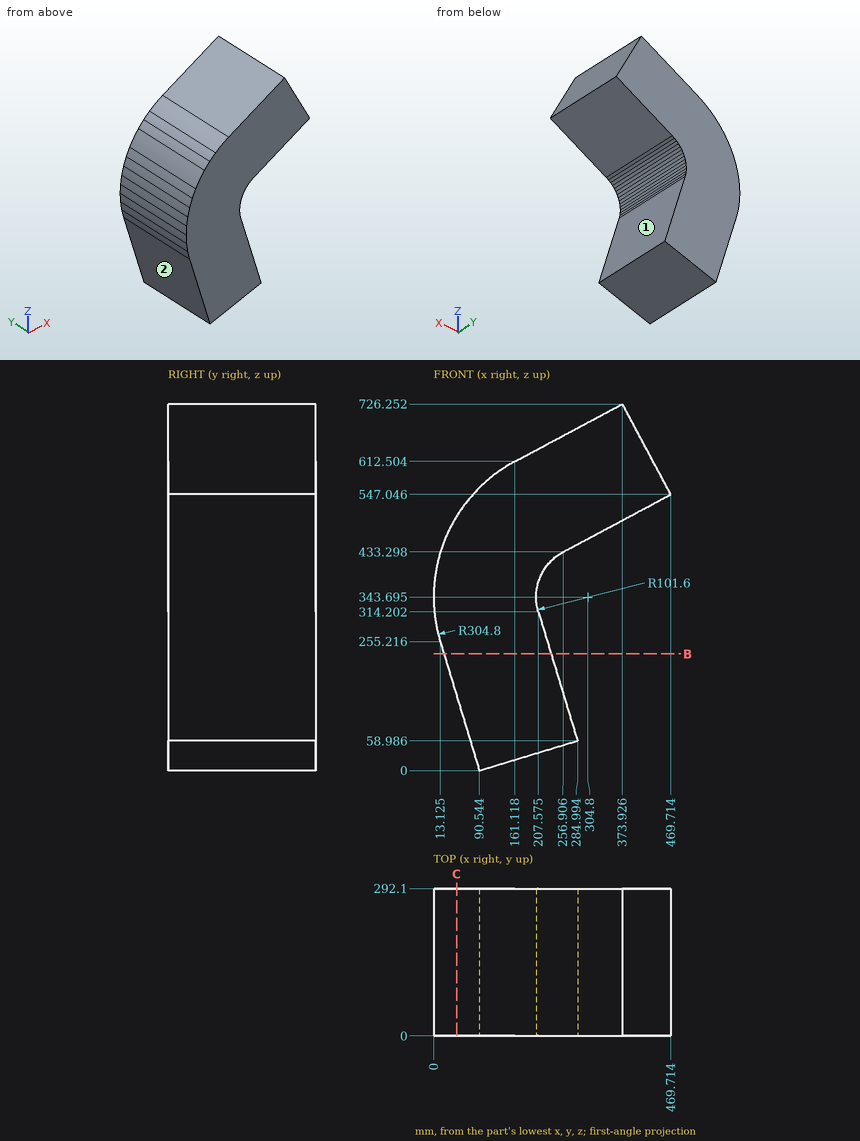
Check sheet for the drawn part. Datum: minimum x, y, z corner. Units: mm. A direction names the side the tool comes from. Round coordinates to 2 decimals unless told otherwise and drop trailing zeros. Loops run counter-clockwise (first coordinate to the right, second up) from the corner with the lowest first, then second, coordinate; pieces in that order, holes last. Notation, with made-up numbers: (88, 21) -> (114, 21) arc R25 ccw to (114, 39) -> close; hole circle Ø5 at (31, -30.75). An arc over 180 degrees is marked (long way). Put each result on its own line as item: value. Start each with the question number.
1. Access from +Z, -Z, +X, -X, +Y, -Y to the whole of each face (thin tool, end or side, straight path). Record for the marked faces 1 and 2.
2. Section check C-C (x = 45.5). Enter the section's corners in (y, z), plus the area to 3 significant figures.
3. Scan lines: probe 1 along X at (y, z) = (205, 216) (1 decimal); probe 2 along X at (y, z) = (121, 127.5); probe 3 along Z at (x, y) = (165.5, 125.5) (1 decimal). Record each from-to range of solid material in increasing order.
4. Section check B-B (z = 231). Enter the section's corners in (x, y).
5. Gauge pin test, flat ends, axial feed: pin 1 (4 mm diameter, centred on y = 196.5, z = 333, fed in from +X); pin 2 (1 mm diameter, centred on y = 151.5, z = 616.5, fed in from +X); pin 3 (1.5 mm diameter, centred on y = 115, z = 345, fed in from -X). Record the tip position at first contact, or that the pin passes through.
Findings:
1. face 1: +X, +Y, -Y
1. face 2: -Z, -X, +Y, -Y
2. outline: (0, 148.49) -> (292.1, 148.49) -> (292.1, 503.9) -> (0, 503.9) -> close
2. area: 104,000 mm^2
3. probe 1: x = 25 to 237.4
3. probe 2: x = 51.87 to 264.21
3. probe 3: z = 22.7 to 614.8
4. outline: (20.47, 0) -> (232.81, 0) -> (232.81, 292.1) -> (20.47, 292.1) -> close
5. pin 1: stops at x = 204
5. pin 2: stops at x = 432.86
5. pin 3: stops at x = 0
